```python
from build123d import *

# Parameters (mm, degrees)
F1_DEPTH = 76.2
F2_R     = 7.15
F3_DEPTH = 9.501
F4_R     = 5
F5_R     = 5


with BuildPart() as f1:
    # F0 (on Top) → F1 (new body)
    with BuildSketch(Plane.XY):
        Polygon((0, 9.5), (0, 0), (681.5, 0), (681.5, 250.8), (672, 250.8), (672, 9.5), align=None)
    extrude(amount=F1_DEPTH)

    # F2 (on face) → F3 (cut, through all)
    with BuildSketch(Plane(origin=(0, 9.5, 0), x_dir=(-1, 0, 0), z_dir=(0, 1, 0))):
        with Locations((-38.1, 38.1)):
            Circle(F2_R)
        with Locations((-82.6, 38.1)):
            Circle(F2_R)
        with Locations((-189, 38.1)):
            Circle(F2_R)
    extrude(amount=-F3_DEPTH, mode=Mode.SUBTRACT)

    # F4
    f4_edges = [f1.edges().sort_by_distance(p)[0] for p in [
        (681.5, 0, 38.1),
    ]]
    fillet(f4_edges, radius=F4_R)

    # F5
    f5_edges = [f1.edges().sort_by_distance(p)[0] for p in [
        (672, 9.5, 38.1),
    ]]
    fillet(f5_edges, radius=F5_R)


solid = f1.part
```
Can you work these out from the model? Positions are in its coordinate system, mm. A direction names the side the tool comes from. Give positions to 0.01 mm unless a question says otherwise; leave off trailing zeros. Order: outer loops, then holes, each group sorted by start corner. A loop starts at its lowest first (then second) coordinate and runs counter-clockwise, first axis right, second up. Notation, with made-up numbers: (21, -13.5) - (45, -13.5) arc R12 cw to (45, 9.5) - close; hole circle Ø1 at (38, -1.75). An arc over 180 degrees is marked (long way). Use a Markdown table: item, result. Add a question column.
Q1. Please list where these lines run through material, in increasing order: line 1 along X through (y, z) = (6, 38); line 2 along Z through (x, y) = (189, 5.75); line 3 along Y through (x, z) = (46.5, 43.5).
Q2. I'm going to push flat-ended pins straight in: pin 1 (3 mm diameter, centred on y = 160, z = 67.5, fed in from -X); pin 2 (18.5 mm diameter, centred on x = 82.6, z = 38.1, fed in from -Y); pin 3 (8.5 mm diameter, centred on x = 189, z = 38.1, fed in from +Y); pin 4 (18.5 mm diameter, centred on x = 38.1, z = 38.1, fed in from +Y). Where does each tip first touch, or does it pass through?
Q3. If we mould it in two halves opening along Z, with no side actions, what happens to faces 1 (the cylindrical face through (34.801, 4.816, 31.757)), 2 (the flat face through (339, 5, 76.2)), 3 (the flat face through (338, 9.5, 38))? For each: released by +Z, released by -Z, zero draft, split by the parting line, or undercut.
Q4. On a 3-axis mill with a long thin cutter (end or side, diameter ignored), from which of +Z, -Z, +X, -X, +Y, -Y can I reach the whole of each face in a straight line? I mean faces 4 (the cylindrical face through (75.995, 4.816, 35.362)), 5 (the flat face through (672, 134, 38)). Say none if no direction works.
Q5. If we section it at D-D on y = 217: Write out the boundary of the cut face in (x, z).
Q6. If we section it at A-A on x = 82.6: Write out the boundary of the cut face in (y, z).
Q7. If we section it at B-B on z = 38.1: Write out the boundary of the cut face in (x, y), plus the area to 3 significant figures.
Q8. If we section it at C-C on z = 66.5: Write out the boundary of the cut face in (x, y).
Answers follow:
| question | item | result |
|---|---|---|
| 1 | line 1 | x = 0 to 30.95, 45.25 to 75.45, 89.75 to 181.85, 196.15 to 681.5 |
| 1 | line 2 | z = 0 to 30.95, 45.25 to 76.2 |
| 1 | line 3 | y = 0 to 9.5 |
| 2 | pin 1 | stops at x = 672 |
| 2 | pin 2 | stops at y = 0 |
| 2 | pin 3 | passes through |
| 2 | pin 4 | stops at y = 9.5 |
| 3 | face 1 | undercut |
| 3 | face 2 | released by +Z |
| 3 | face 3 | zero draft |
| 4 | face 4 | +Y, -Y |
| 4 | face 5 | +Z, -Z, -X, +Y |
| 5 | outline | (672, 0) - (681.5, 0) - (681.5, 76.2) - (672, 76.2) - close |
| 6 | outline | (0, 0) - (9.5, 0) - (9.5, 30.95) - (0, 30.95) - close; (0, 45.25) - (9.5, 45.25) - (9.5, 76.2) - (0, 76.2) - close |
| 7 | outline | (0, 0) - (30.95, 0) - (30.95, 9.5) - (0, 9.5) - close; (45.25, 0) - (75.45, 0) - (75.45, 9.5) - (45.25, 9.5) - close; (89.75, 0) - (181.85, 0) - (181.85, 9.5) - (89.75, 9.5) - close; (196.15, 0) - (676.5, 0) arc R5 ccw to (681.5, 5) - (681.5, 250.8) - (672, 250.8) - (672, 14.5) arc R5 cw to (667, 9.5) - (196.15, 9.5) - close |
| 7 | area | 8,360 mm^2 |
| 8 | outline | (0, 0) - (676.5, 0) arc R5 ccw to (681.5, 5) - (681.5, 250.8) - (672, 250.8) - (672, 14.5) arc R5 cw to (667, 9.5) - (0, 9.5) - close |
